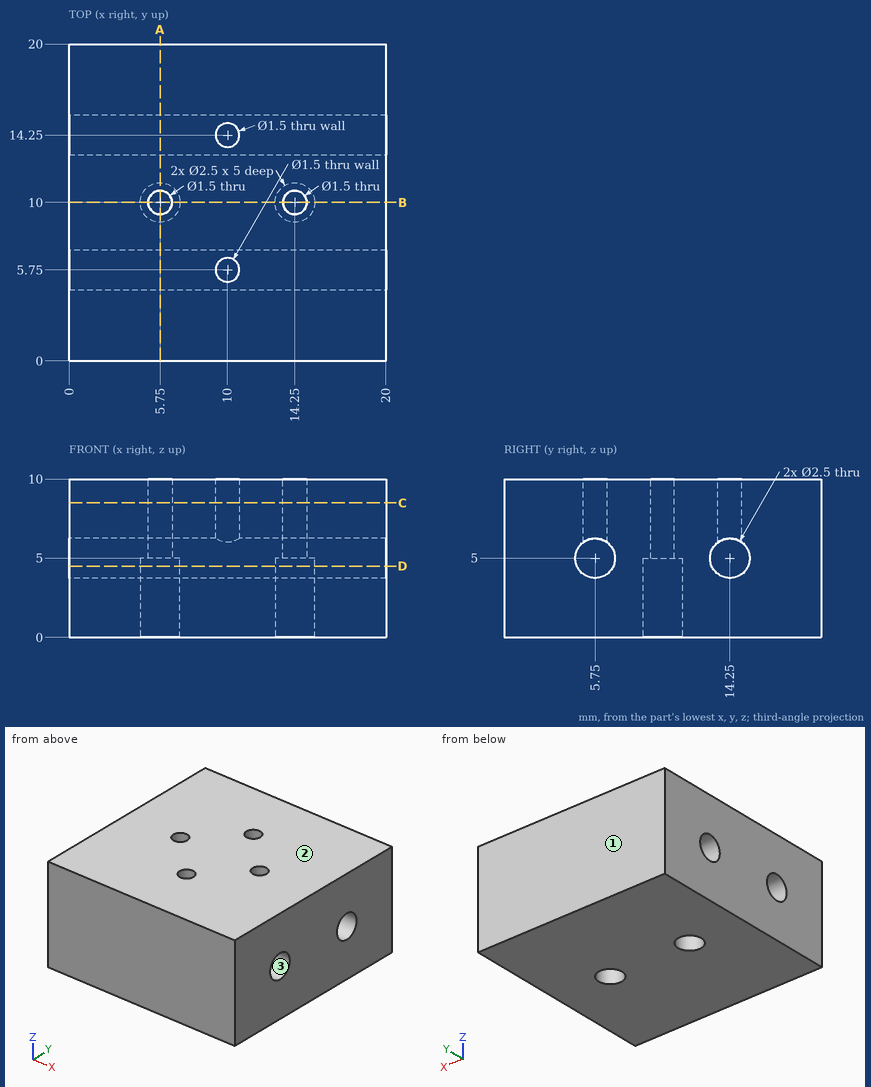
Geometry: see drawing. Coordinates: mm, zero at the bounding-box minimum. Round coordinates to 2 decimals unless told otherwise and drop trailing zeros. Write each loop counter-clockwise with the first axis right and the second up, starting at its lowest first coordinate (ties: lowest second). Pieces come first, ordered by that corner, then holes.
Item 1: Section query D-D (z = 4.5). Return loops of the section in (x, y), plus the area to 3 significant figures.
Item 2: Pin query (flat end, axial travel): P1, Ø3, axis at x = 13, y = 11, coming from the -Z side; P2, Ø1.7, axis at x = 14.25, y = 10, coming from the -Z side; P3, Ø0.9, axis at x = 10, y = 14.25, coming from the +Z side. Return the tip coordinate at first contact, or that it passes through.
Item 3: Mould query, pull axis Z, two halves, no side actions, for the marked faces 1, 2 and 3. Classes: +Z half, -Z half, draft (parallel to the pull), parting line (faces both ways), or undercut.
Item 4: Section query C-C (z = 8.5). Return loops of the section in (x, y), plus the area to 3 significant figures.
Item 5: Section query B-B (y = 10). Return loops of the section in (x, z), plus the area to 3 significant figures.
Item 6: Section query A-A (x = 5.75). Return loops of the section in (y, z), plus the area to 3 significant figures.
Item 7: Material intervals for L1, parallel to Y at x = 10, z = 8.25; L2, parallel to X at y = 10, z = 4.05; L3, parallel to Y at x = 5.75, z = 2.1, sorted ascending.
Completed:
1. outline: (0, 0) - (20, 0) - (20, 4.6) - (0, 4.6) - close; (0, 6.9) - (20, 6.9) - (20, 13.1) - (0, 13.1) - close; (0, 15.4) - (20, 15.4) - (20, 20) - (0, 20) - close; hole circle Ø2.5 at (5.75, 10); hole circle Ø2.5 at (14.25, 10)
1. area: 299 mm2
2. P1: stops at z = 0
2. P2: stops at z = 5
2. P3: stops at z = 3.83
3. face 1: draft
3. face 2: +Z half
3. face 3: undercut
4. outline: (0, 0) - (20, 0) - (20, 20) - (0, 20) - close; hole circle Ø1.5 at (5.75, 10); hole circle Ø1.5 at (10, 5.75); hole circle Ø1.5 at (10, 14.25); hole circle Ø1.5 at (14.25, 10)
4. area: 393 mm2
5. outline: (0, 0) - (4.5, 0) - (4.5, 5) - (5, 5) - (5, 10) - (0, 10) - close; (6.5, 5) - (7, 5) - (7, 0) - (13, 0) - (13, 5) - (13.5, 5) - (13.5, 10) - (6.5, 10) - close; (15, 5) - (15.5, 5) - (15.5, 0) - (20, 0) - (20, 10) - (15, 10) - close
5. area: 160 mm2
6. outline: (0, 0) - (8.75, 0) - (8.75, 5) - (9.25, 5) - (9.25, 10) - (0, 10) - close; (10.75, 5) - (11.25, 5) - (11.25, 0) - (20, 0) - (20, 10) - (10.75, 10) - close; hole circle Ø2.5 at (5.75, 5); hole circle Ø2.5 at (14.25, 5)
6. area: 170 mm2
7. L1: y = 0 to 5, 6.5 to 13.5, 15 to 20
7. L2: x = 0 to 4.5, 7 to 13, 15.5 to 20
7. L3: y = 0 to 8.75, 11.25 to 20
